Can you work these out from the drawing? Everything is in mm from the part's minimum corner. A direction names the side the tool comes from. Give positions to 0.01 mm unless a question says otherwise; leave off trailing zeros. Loops run counter-clockwise (first coordinate to the right, second up) from the corner with the lowest first, then second, coordinate; pieces in that order, holes last. Notation, with made-up numbers: (58.5, 22) - (96.5, 22) arc R28 ccw to (96.5, 57) - close; hole circle Ø6 at (42, -34). An arc over 180 degrees is marked (long way). Answer in a Markdown table with one row per item.
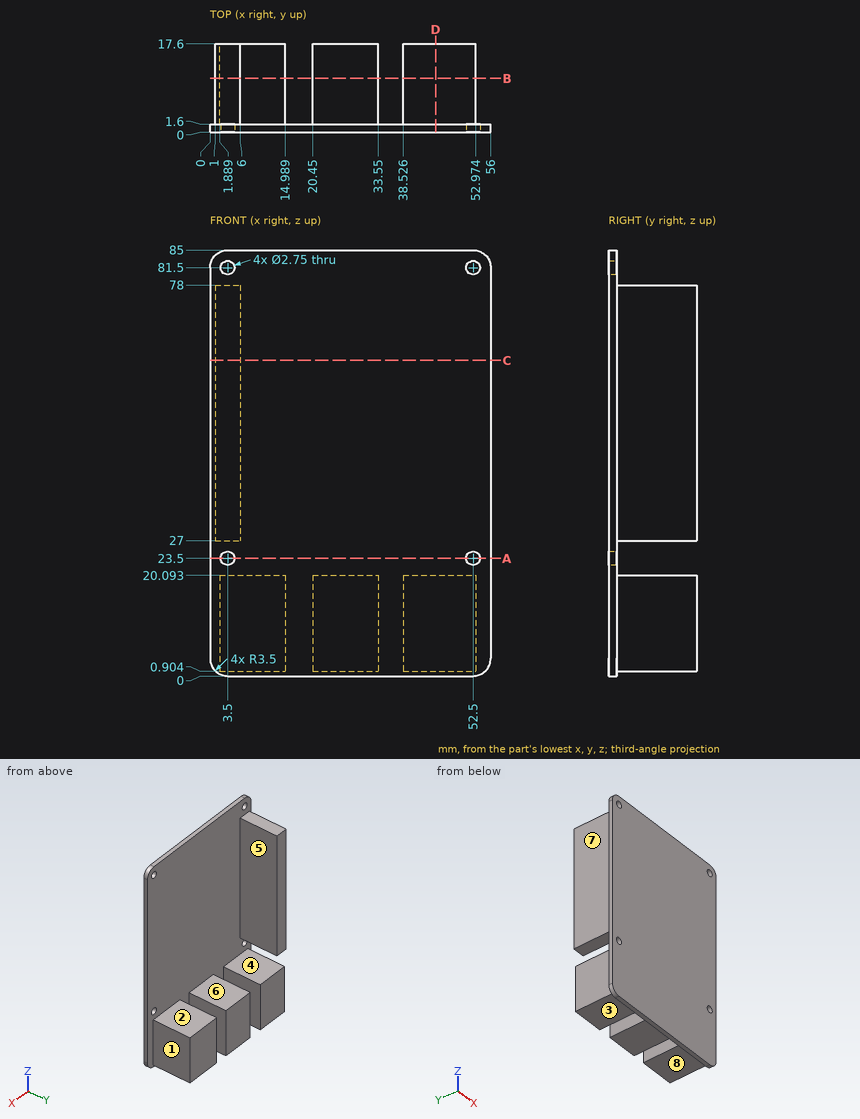
Q1. Imagine slicing it at D-D, the plane x = 45. Write out the boundary of the cut face in (y, z), and give its area (3 significant figures).
Checked values:
| item | result |
|---|---|
| outline | (0, 0) - (1.6, 0) - (1.6, 0.9) - (17.6, 0.9) - (17.6, 20.09) - (1.6, 20.09) - (1.6, 85) - (0, 85) - close |
| area | 443 mm² |
Q2. If we mould it in two halves opening along Z, with no side actions, what happens to the marked faces 1, 2, 3 and 4? For each: released by +Z, released by -Z, zero draft, split by the parting line, or undercut.
Checked values:
| item | result |
|---|---|
| face 1 | zero draft |
| face 2 | released by +Z |
| face 3 | released by -Z |
| face 4 | undercut |
Q3. If I drill on line 1 (X direction, y = 0.6, z = 23.5) (1 decimal); line 2 (Y direction, x = 32.5, z = 40.5); line 3 (X direction, y = 16, z = 49), over which ranges is the centre line in solid material (lowest first)? Write a range as [from, to].
Checked values:
| item | result |
|---|---|
| line 1 | x = [0, 2.1], [4.9, 51.1], [53.9, 56] |
| line 2 | y = [0, 1.6] |
| line 3 | x = [1, 6] |
Q4. For pin 1 (5 mm diameter, centred on y = 13, z = 15, fed in from -X); pin 2 (10.5 mm diameter, centred on x = 28, y = 12.5, fed in from -Z); pin 3 (6 mm diameter, centred on y = 5.5, z = 35, fed in from -X), each with a flat end and sliding along its axis, tell me the tip position at first contact or that it passes through.
Checked values:
| item | result |
|---|---|
| pin 1 | stops at x = 1.89 |
| pin 2 | stops at z = 0.9 |
| pin 3 | stops at x = 1 |
Q5. Imagine slicing it at C-C, the plane z = 63. Write out the boundary of the cut face in (x, y).
Checked values:
| item | result |
|---|---|
| outline | (0, 0) - (56, 0) - (56, 1.6) - (6, 1.6) - (6, 17.6) - (1, 17.6) - (1, 1.6) - (0, 1.6) - close |
Q6. Imagine slicing it at B-B, the plane y = 10.75. Count the separate pieces of the cut face and the enclosed holes in it, and give its area (4 significant figures).
Checked values:
| item | result |
|---|---|
| separate pieces | 4 |
| enclosed holes | 0 |
| area | 1,035 mm² |
Q7. Imagine slicing it at A-A, the plane z = 23.5. Write out the boundary of the cut face in (x, y) (1 decimal).
Checked values:
| item | result |
|---|---|
| outline | (0, 0) - (2.1, 0) - (2.1, 1.6) - (0, 1.6) - close; (4.9, 0) - (51.1, 0) - (51.1, 1.6) - (4.9, 1.6) - close; (53.9, 0) - (56, 0) - (56, 1.6) - (53.9, 1.6) - close |
Q8. On a 3-axis mill with a long thin cutter (end or side, diameter ignored), from which of +Z, -Z, +X, -X, +Y, -Y can I reach the whole of each face in a straight line? I mean the marked faces 5, 6, 7 and 8. Say none if no direction works.
Checked values:
| item | result |
|---|---|
| face 5 | +Z, +X, +Y |
| face 6 | +Z, +X, -X, +Y |
| face 7 | +Z, -Z, -X, +Y |
| face 8 | -Z, +X, -X, +Y |
